from build123d import *

# Parameters (mm, degrees)
SKETCH1_W                = 140
SKETCH1_H                = 60
BOSS_EXTRUDE1_DEPTH      = 5
SKETCH2_R                = 7.45
SKETCH2_R_2              = 6
CUT_EXTRUDE1_DEPTH       = 5
BOSS_EXTRUDE3_DEPTH      = 100
BOSS_EXTRUDE3_DEPTH_BACK = 5
SKETCH3_R                = 7.45
SKETCH4_R                = 17.5
BOSS_EXTRUDE4_DEPTH      = 28


with BuildPart() as part:
    # Sketch1 → Boss-Extrude1 (new body)
    with BuildSketch(Plane.XY):
        Rectangle(SKETCH1_W, SKETCH1_H)
    extrude(amount=BOSS_EXTRUDE1_DEPTH)

    # Sketch2 → Cut-Extrude1 (cut)
    with BuildSketch(Plane.XY.offset(5)):
        Circle(SKETCH2_R)
        with Locations((-45, 15)):
            Circle(SKETCH2_R_2)
        with Locations((45, 15)):
            Circle(SKETCH2_R_2)
        with Locations((-45, -15)):
            Circle(SKETCH2_R_2)
        with Locations((45, -15)):
            Circle(SKETCH2_R_2)
    extrude(amount=-CUT_EXTRUDE1_DEPTH, mode=Mode.SUBTRACT)

    # Sketch3 → Boss-Extrude3 (add, two sides: drawn at the far end of the back side and taken through both)
    with BuildSketch(Plane.XY.offset(5).offset(-BOSS_EXTRUDE3_DEPTH_BACK)):
        Circle(SKETCH3_R)
    extrude(amount=BOSS_EXTRUDE3_DEPTH + BOSS_EXTRUDE3_DEPTH_BACK)

    # Sketch4 → Boss-Extrude4 (add)
    with BuildSketch(Plane.XY.offset(5)):
        Circle(SKETCH4_R)
    extrude(amount=BOSS_EXTRUDE4_DEPTH)


solid = part.part
Build history of the part. All positions in model axes, mm. A direction names the side the tool comes from. Round coordinates to 2 decimals unless told otherwise and drop trailing zeros. Write each loop counter-clockwise with the first axis right and the second up, starting at its lowest first coordinate (ties: lowest second). Pieces come first, ordered by that corner, then holes. Notation, with made-up numbers: M 15,55.25 L 52,55.25 A26 cw 52,78.25 Z; hole C -17,79 d5. An arc over 180 degrees is marked long. Answer in a Markdown table with one row per item.
1. Saw through at A-A (x = 45). List the corners of the cut face in (y, z), and give its area (3 significant figures).
Geometry check:
| item | result |
|---|---|
| outline | M -30,0 L -21,0 L -21,5 L -30,5 Z; M -9,0 L 9,0 L 9,5 L -9,5 Z; M 21,0 L 30,0 L 30,5 L 21,5 Z |
| area | 180 mm2 |
2. Saw through at D-D (y = 0). List the corners of the cut face in (x, z), and give its area (3 significant figures).
Geometry check:
| item | result |
|---|---|
| outline | M -70,0 L 70,0 L 70,5 L 17.5,5 L 17.5,33 L 7.45,33 L 7.45,105 L -7.45,105 L -7.45,33 L -17.5,33 L -17.5,5 L -70,5 Z |
| area | 2,750 mm2 |
3. Flat gauge pins, fed straight in: P1, Ø2, axis at x = -30, y = 6, coming from the +Z side; P2, Ø3, axis at x = 16.5, y = -22.5, coming from the -Z side; P3, Ø5, axis at y = -7.5, z = 82.5, coming from the +X side; P4, Ø6, axis at x = -19, z = 27, coming from the -Y side. Where does each tip first touch, or does it go through?
Geometry check:
| item | result |
|---|---|
| P1 | z = 5 |
| P2 | z = 0 |
| P3 | x = 5.52 |
| P4 | y = -7.09 |
4. Which spindle directions (+Z, -Z, +X, -X, +Y, -Y) get a long thin tool onto all of the face, cutting with end or side? Do faces 1 (the face through (0, -8, 33)), 2 (the face through (-1, 0, 0)). Say none if no direction does.
Geometry check:
| item | result |
|---|---|
| face 1 | +Z |
| face 2 | -Z, +X, -X, +Y, -Y |
5. Saw through at C-C (x = 0). List the corners of the cut face in (y, z), and give its area (3 significant figures).
Geometry check:
| item | result |
|---|---|
| outline | M -30,0 L 30,0 L 30,5 L 17.5,5 L 17.5,33 L 7.45,33 L 7.45,105 L -7.45,105 L -7.45,33 L -17.5,33 L -17.5,5 L -30,5 Z |
| area | 2,350 mm2 |
6. Saw through at B-B (y = -15). List the corners of the cut face in (x, z), and give its area (3 significant figures).
Geometry check:
| item | result |
|---|---|
| outline | M -70,0 L -51,0 L -51,5 L -70,5 Z; M -39,0 L 39,0 L 39,5 L 9.01,5 L 9.01,33 L -9.01,33 L -9.01,5 L -39,5 Z; M 51,0 L 70,0 L 70,5 L 51,5 Z |
| area | 1,080 mm2 |
7. Probe L1, parallel to Y at x = -45, z = 3; L2, parallel to Z at x = -11.5, y = 1; L3, parallel to Z at x = 38, y = 26.5. List the from-to ranges inside material, lowest first. Write a range as [from, to].
Geometry check:
| item | result |
|---|---|
| L1 | [-30, -21], [-9, 9], [21, 30] |
| L2 | [0, 33] |
| L3 | [0, 5] |
